Could you check a few things on this model? Use its own coordinates, in mm. Round coordinates to 2 decimals unless told otherwise and drop trailing zeros. Loops run counter-clockwise (first coordinate to the right, second up) from the corner with the lowest first, then second, coordinate; pieces in that order, holes last. Notation, with made-up numbers: (14, 63.25) -> (37, 63.25) arc R10 ccw to (37, 67.25) -> close; hole circle Ø11 at (55, 49.5). An arc over 180 degrees is marked (long way). Put each result on its own line as item: value. Start each with the question number.
1. Imagine slicing it at D-D, the plane y = 538. Please give me the cut outline in (x, z).
2. I need wall thicknesses on line 1 (Z direction, x = -5243, y = 830); line 2 (Y direction, x = -5085.5, z = 2141); line 3 (Z direction, x = -5369, y = 955). Which ranges of each line are inside material? Lowest first, please. Write a range as [from, to].
3. I'm going to push flat-ended pins straight in: P1, Ø1, axis at y = 616, z = 2312.5, coming from the -X side; P2, Ø8, axis at y = 890.5, z = 2118.5, coming from the +X side; P3, Ø10, axis at x = -5594, y = 973, coming from the +Z side. Where does each tip first touch, or does it pass through?
4. Imagine slicing it at C-C, the plane z = 2155. Please give me the cut outline in (x, y).
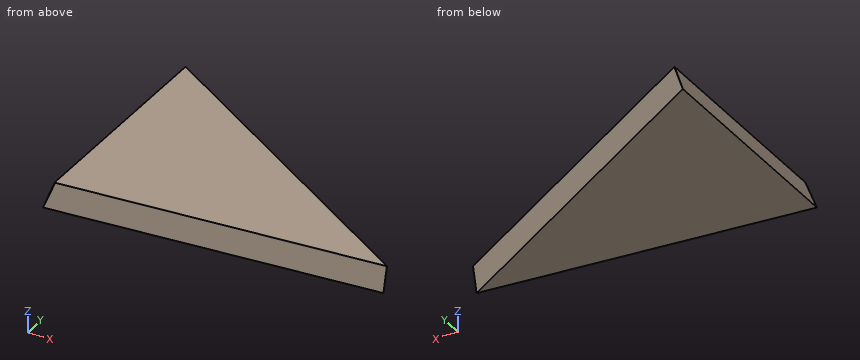
```python
from build123d import *

# Parameters (mm, degrees)
BOSS_EXTRUDE1_DEPTH = 70
CHAMFER1_SIZE2      = 4.18941816
CHAMFER1_SIZE       = 70
CHAMFER2_SIZE       = 6.666257335
CHAMFER2_SIZE_2     = 70
CUT_EXTRUDE1_DEPTH  = 10
CUT_EXTRUDE2_DEPTH  = 10
SKETCH4_W           = 287.422720902
SKETCH4_H           = 893.518312169
CUT_EXTRUDE3_DEPTH  = 10


# Some blends are built 0.0001 mm under size
with BuildPart() as part:
    # Sketch1 → Boss-Extrude1 (new body)
    with BuildSketch(Plane(origin=(231.948409601, 267.750179411, 1224.939426156), x_dir=(0.9836670614243895, -0.018848869033306223, -0.17900791157061058), z_dir=(0.17900684147746093, 0.20663786272562784, 0.9619029807586875))):
        Polygon((-6114.579700227, 916.675736405), (-6017.047344534, 65.828535372), (-5261.298623968, 468.69003921), align=None)
    extrude(amount=BOSS_EXTRUDE1_DEPTH)

    # Chamfer1
    chamfer1_edges = [part.edges().sort_by_distance(p)[0] for p in [
        (-5363.622839272, 1067.033331681, 2167.324875996),
    ]]
    chamfer1_side = [part.faces().sort_by_distance(p)[0] for p in [
        (-5363.637837962, 1067.016017832, 2167.24427972),
    ]]
    chamfer(chamfer1_edges, length=CHAMFER1_SIZE - 0.0001, length2=CHAMFER1_SIZE2 - 0.0001, reference=chamfer1_side[0])  # a hair under: the kernel refuses the full size

    # Chamfer2
    # the kernel refuses this chamfer: 70, 6.666257335 mm, written as the material it takes off along each edge
    with BuildSketch(Plane(origin=(-5831.876326045, 379.315966254, 2402.202019272), x_dir=(-0.37796472427930605, 0.8862370425990936, 0.267818168774414), z_dir=(0.8591676949824762, 0.4435312395800335, -0.255168398151295))) as chamfer2_piece_1:
        Polygon((CHAMFER2_SIZE * 0.92779638202, -CHAMFER2_SIZE * 0.373086951719), (-CHAMFER2_SIZE_2 * 0.373086951713, -CHAMFER2_SIZE_2 * 0.927796382005), (0, 0), align=None)
    extrude(amount=1215.290815937, mode=Mode.SUBTRACT)
    with BuildSketch(Plane(origin=(-5810.651127776, 1466.498755071, 2164.701368848), x_dir=(-0.1825618043812556, -0.20697447902057858, -0.9611621885068203), z_dir=(0.13076019619656676, -0.9740181607293223, 0.184906445696475))) as chamfer2_piece_2:
        Polygon((CHAMFER2_SIZE_2 * 0.999993350078, CHAMFER2_SIZE_2 * 0.00364688918346), (-CHAMFER2_SIZE * 0.00364688918357, CHAMFER2_SIZE * 0.999993350094), (0, 0), align=None)
    extrude(amount=1215.290815937, mode=Mode.SUBTRACT)

    # Sketch2 → Cut-Extrude1 (cut)
    with BuildSketch(Plane(origin=(-1155.31957462, -2341.467412338, 1286.584724908), x_dir=(0.9178561698216066, -0.3478582739738773, 0.1911404529353356), z_dir=(-0.39691315362483304, -0.8044174401239645, 0.4420096497860625))):
        Polygon((-4919.324722598, 2288.84825515), (-4917.313875734, 2288.259664395), (-4938.404193289, 2220.173354917), align=None)
    extrude(amount=CUT_EXTRUDE1_DEPTH, mode=Mode.SUBTRACT)

    # Sketch3 → Cut-Extrude2 (cut)
    with BuildSketch(Plane(origin=(-4820.811559407, -663.513212633, 188.265036569), x_dir=(-0.038297874166628845, -0.005271134374818051, -0.9992524645837606), z_dir=(0.9899202066384638, 0.1362478347188717, -0.03865891906507896))):
        Polygon((-2346.226398356, 930.896979041), (-1894.241052266, 2187.396241778), (-1814.981817773, 1495.770397412), align=None)
    extrude(amount=CUT_EXTRUDE2_DEPTH, mode=Mode.SUBTRACT)

    # Sketch4 → Cut-Extrude3 (cut)
    with BuildSketch(Plane(origin=(-1646.015630594, 3413.926203867, 236.836708654), x_dir=(0.9011742428578655, 0.43241771341973545, 0.029998418798336916), z_dir=(-0.43345701518092067, 0.8990134934757245, 0.06236789670191585))):
        with Locations((-4715.577586911, -1688.111490452)):
            Rectangle(SKETCH4_W, SKETCH4_H)
    extrude(amount=CUT_EXTRUDE3_DEPTH, mode=Mode.SUBTRACT)


solid = part.part
```
Entries:
1. outline: (-5700.47, 2270.89) -> (-5509, 2235.25) -> (-5538.95, 2313.6) -> (-5679.42, 2339.74) -> close
2. line 1: [2123.02, 2195.8]
2. line 2: [763.64, 911.6]
2. line 3: [2119.62, 2192.39]
3. P1: x = -5693.85
3. P2: x = -5047.32
3. P3: z = 2231.82
4. outline: (-5792.57, 1281.6) -> (-5782.43, 1148.45) -> (-5238.78, 677.5) -> (-5004.93, 813.68) -> (-5176.11, 961.97) -> (-5792.35, 1281.71) -> close
